```python
from build123d import *

# Parameters (mm, degrees)
SALIENTE_EXTRUIR1_DEPTH = 2
CROQUIS2_R              = 1.5
CORTAR_EXTRUIR1_DEPTH   = 2
CHAFL_N1_SIZE           = 1
CROQUIS3_R              = 1.6
CORTAR_EXTRUIR2_DEPTH   = 2
CROQUIS4_R              = 7
CROQUIS4_W              = 9.2
CROQUIS4_H              = 15.1
CORTAR_EXTRUIR3_DEPTH   = 2
REDONDEO1_R             = 1


with BuildPart() as part:
    # Croquis1 → Saliente-Extruir1 (new body)
    with BuildSketch(Plane(origin=(0, 0, 0), x_dir=(1, 0, 0), z_dir=(0, 1, 0))):
        with BuildLine():
            Line((-65, -40), (65, -40))
            ThreePointArc((65, -40), (68.535533906, -38.535533906), (70, -35))
            Line((70, -35), (70, 35))
            ThreePointArc((70, 35), (68.535533906, 38.535533906), (65, 40))
            Line((65, 40), (-65, 40))
            ThreePointArc((-65, 40), (-68.535533906, 38.535533906), (-70, 35))
            Line((-70, 35), (-70, -35))
            ThreePointArc((-70, -35), (-68.535533906, -38.535533906), (-65, -40))
        make_face()
    extrude(amount=SALIENTE_EXTRUIR1_DEPTH)

    # Croquis2 → Cortar-Extruir1 (cut)
    with BuildSketch(Plane(origin=(0, 2, 0), x_dir=(1, 0, 0), z_dir=(0, 1, 0))):
        with Locations(Location((65, 35, 0), (0, 0, 270))):
            Circle(CROQUIS2_R)
        with Locations(Location((65, -35, 0), (0, 0, 90))):
            Circle(CROQUIS2_R)
        with Locations(Location((-65, -35, 0), (0, 0, 270))):
            Circle(CROQUIS2_R)
        with Locations(Location((-65, 35, 0), (0, 0, 90))):
            Circle(CROQUIS2_R)
    extrude(amount=-CORTAR_EXTRUIR1_DEPTH, mode=Mode.SUBTRACT)

    # Chaflán1
    chafl_n1_edges = [part.edges().sort_by_distance(p)[0] for p in [
        (-65, 2, -33.5),
        (-65, 2, 33.5),
        (65, 2, 36.5),
        (65, 2, -36.5),
    ]]
    chamfer(chafl_n1_edges, length=CHAFL_N1_SIZE)

    # Croquis3 → Cortar-Extruir2 (cut)
    with BuildSketch(Plane(origin=(0, 2, 0), x_dir=(1, 0, 0), z_dir=(0, 1, 0))):
        with Locations(Location((4, 7.5, 0), (0, 0, 270))):
            Circle(CROQUIS3_R)
        with Locations(Location((4, -7.5, 0), (0, 0, 270))):
            Circle(CROQUIS3_R)
        with BuildLine():
            Line((-10.5, -10), (-10.5, 10))
            ThreePointArc((-10.5, 10), (-8, 12.5), (-5.5, 10))
            Line((-5.5, 10), (-5.5, -10))
            ThreePointArc((-5.5, -10), (-8, -12.5), (-10.5, -10))
        make_face()
    extrude(amount=-CORTAR_EXTRUIR2_DEPTH, mode=Mode.SUBTRACT)

    # Croquis4 → Cortar-Extruir3 (cut)
    with BuildSketch(Plane(origin=(0, 2, 0), x_dir=(1, 0, 0), z_dir=(0, 1, 0))):
        with Locations(Location((-40, 0, 0), (0, 0, 270))):
            Circle(CROQUIS4_R)
        with Locations((50, 0)):
            Rectangle(CROQUIS4_W, CROQUIS4_H)
    extrude(amount=-CORTAR_EXTRUIR3_DEPTH, mode=Mode.SUBTRACT)

    # Redondeo1
    redondeo1_edges = [part.edges().sort_by_distance(p)[0] for p in [
        (68.535533906, 2, 38.535533906),
        (70, 2, 0),
        (68.535533906, 2, -38.535533906),
        (0, 2, -40),
        (-68.535533906, 2, -38.535533906),
        (-70, 2, 0),
        (-68.535533906, 2, 38.535533906),
        (0, 2, 40),
    ]]
    fillet(redondeo1_edges, radius=REDONDEO1_R)


solid = part.part
```
Verification items for the finished model (mm, model axes). A direction names the side the tool comes from. Give positions to 0.01 mm unless a question says otherwise; leave off trailing zeros. Order: outer loops, then holes, each group sorted by start corner. A loop starts at its lowest first (then second) coordinate and runs counter-clockwise, first axis right, second up. Notation, with made-up numbers: M 4,77.5 L 13,77.5 A12 cw 13,83.5 Z; hole C -9,14.25 d10. An arc over 180 degrees is marked long. Return JSON: item names as keys, results as strings. Group by question number.
1) Access from +Z, -Z, +X, -X, +Y, -Y to the whole of each face (thin tool, end or side, straight path). Record for faces 1 (the face through (-7.9, 1, 12.5)), 2 (the face through (-68.57, 0.49, 38.5)).
2) Section check A-A on x = -8. Record the cut outline in (y, z).
3) Mould release check, pull along Z, two halves, no side actions. Record for faces 3 (the face through (-33.06, 1.01, -0.91)), 4 (the face through (-1, 2, -1)), 5 (the face through (-68.5, 0.49, -38.57)): pulls with the +Z half, pulls with the -Z half, needs draft (parallel to the pull), parting line crosses it, or undercut.
4) Scan lines: line 1 (Z direction, x = -65, y = 0.3); line 2 (X direction, y = 1, z = 0); line 3 (X direction, y = 0.85, z = 7.5). Record each from-to range of solid material in increasing order.
5) Section check C-C on z = 3.5. Record the cut outline in (x, y).
6) Section check B-B on y = 0.4. Give the number of separate pieces and of enclosed holes in the cut face, and give its area (3 significant figures).
7) Go/stop test with flat-tipped pins: pin 1 Ø2.5 at (x, z) = (-65, -35) entering from -Y; pin 2 Ø0.6 at (y, z) = (1.5, -1) entering from +X. Record where each tip stops, or that it passes through.
Answer block:
{
 "1": {"face 1": "+Y, -Y", "face 2": "+Z, -X, +Y, -Y"},
 "2": {"outline": "M 0,-40 L 1,-40 A1 ccw 2,-39 L 2,-12.5 L 0,-12.5 Z; M 0,12.5 L 2,12.5 L 2,39 A1 ccw 1,40 L 0,40 Z"},
 "3": {"face 3": "undercut", "face 4": "needs draft", "face 5": "pulls with the -Z half"},
 "4": {"line 1": "z = -40 to -36.5, -33.5 to 33.5, 36.5 to 40", "line 2": "x = -70 to -47, -33 to -10.5, -5.5 to 45.4, 54.6 to 70", "line 3": "x = -70 to -10.5, -5.5 to 2.4, 5.6 to 45.4, 54.6 to 70"},
 "5": {"outline": "M -70,0 L -46.06,0 L -46.06,2 L -69,2 A1 ccw -70,1 Z; M -33.94,0 L -10.5,0 L -10.5,2 L -33.94,2 Z; M -5.5,0 L 45.4,0 L 45.4,2 L -5.5,2 Z; M 54.6,0 L 70,0 L 70,1 A1 ccw 69,2 L 54.6,2 Z"},
 "6": {"separate pieces": "1", "enclosed holes": "9", "area": "10,700 mm^2"},
 "7": {"pin 1": "passes through", "pin 2": "stops at x = 69.98"}
}
